from build123d import *

# Parameters (mm, degrees)
CROQUIS2_W                                = 104
CROQUIS2_H                                = 54
SALIENTE_EXTRUIR1_DEPTH                   = 66
CORTAR_EXTRUIR1_DEPTH                     = 36
TALADROS_DE_ESPIGA_DE_16_0MM1_D           = 16
TALADROS_DE_ESPIGA_DE_16_0MM1_DEPTH       = 36
TALADROS_DE_ESPIGA_DE_16_0MM1_CSINK_D     = 16.05
TALADROS_DE_ESPIGA_DE_16_0MM1_CSINK_ANGLE = 90
TALADROS_DE_ESPIGA_DE_16_0MM1_TIP         = 4.806884952
CROQUIS7_W                                = 28
CROQUIS7_H                                = 44
SALIENTE_EXTRUIR2_DEPTH                   = 4
CORTAR_EXTRUIR3_DEPTH                     = 100.879927913
CORTAR_EXTRUIR3_DEPTH_BACK                = 100.879927913
CORTAR_EXTRUIR4_DEPTH                     = 100.879927913
CORTAR_EXTRUIR4_DEPTH_BACK                = 100.879927913
CROQUIS9_R                                = 2
TALADRO_ROSCADO_M102_D                    = 8.5
TALADRO_ROSCADO_M102_DEPTH                = 27.5
TALADRO_ROSCADO_M102_CSINK_D              = 10.05
TALADRO_ROSCADO_M102_CSINK_ANGLE          = 90
TALADRO_ROSCADO_M102_TIP                  = 2.553657631


with BuildPart() as part:
    # Croquis2 → Saliente-Extruir1 (new body)
    with BuildSketch(Plane.XY):
        with Locations((0, 27)):
            Rectangle(CROQUIS2_W, CROQUIS2_H)
    extrude(amount=SALIENTE_EXTRUIR1_DEPTH)

    # Croquis3 → Cortar-Extruir1 (cut)
    with BuildSketch(Plane.XY):
        with BuildLine():
            Line((25, 29), (25, 18))
            Line((25, 18), (52, 18))
            Line((52, 18), (52, 54))
            Line((52, 54), (0, 54))
            ThreePointArc((0, 54), (17.67766953, 46.67766953), (25, 29))
        make_face()
    cortar_extruir1 = extrude(amount=CORTAR_EXTRUIR1_DEPTH, mode=Mode.SUBTRACT)

    # Simetría1: Cortar-Extruir1 across plane
    add(cortar_extruir1.mirror(Plane(origin=(0, 0, 0), x_dir=(0, 0, 1), z_dir=(1, 0, 0))), mode=Mode.SUBTRACT)

    # Taladros de espiga de Ø16.0mm1
    with Locations(Plane(origin=(0, 0, 0), x_dir=(-1, 0, 0), z_dir=(0, 0, -1))):
        with Locations((0, 28)):
            CounterSinkHole(TALADROS_DE_ESPIGA_DE_16_0MM1_D / 2, TALADROS_DE_ESPIGA_DE_16_0MM1_CSINK_D / 2, depth=TALADROS_DE_ESPIGA_DE_16_0MM1_DEPTH, counter_sink_angle=TALADROS_DE_ESPIGA_DE_16_0MM1_CSINK_ANGLE)
            with Locations((0, 0, -(TALADROS_DE_ESPIGA_DE_16_0MM1_DEPTH + TALADROS_DE_ESPIGA_DE_16_0MM1_TIP / 2))):  # 118° drill point
                Cone(0, TALADROS_DE_ESPIGA_DE_16_0MM1_D / 2, TALADROS_DE_ESPIGA_DE_16_0MM1_TIP, mode=Mode.SUBTRACT)

    # Croquis7 → Saliente-Extruir2 (add)
    with BuildSketch(Plane(origin=(0, 0, 0), x_dir=(1, 0, 0), z_dir=(0, 1, 0))):
        with Locations((0, -22)):
            Rectangle(CROQUIS7_W, CROQUIS7_H)
    extrude(amount=-SALIENTE_EXTRUIR2_DEPTH)

    # Croquis8 → Cortar-Extruir3 (cut, two sides: drawn at the far end of the back side and taken through both)
    with BuildSketch(Plane(origin=(0, 0, 0), x_dir=(0, 0, -1), z_dir=(1, 0, 0)).offset(-CORTAR_EXTRUIR3_DEPTH_BACK)):
        Polygon((-44, 0), (-56.494918643, 0), (-66, 0), (-66, 24), (-56, 24), (-56, 4), (-44, 4), align=None)
    extrude(amount=CORTAR_EXTRUIR3_DEPTH + CORTAR_EXTRUIR3_DEPTH_BACK, mode=Mode.SUBTRACT)

    # Croquis9 → Cortar-Extruir4 (cut, two sides: drawn at the far end of the back side and taken through both)
    with BuildSketch(Plane(origin=(0, 0, 0), x_dir=(0, 0, -1), z_dir=(1, 0, 0)).offset(-CORTAR_EXTRUIR4_DEPTH_BACK)):
        with Locations((-18, 29)):
            Circle(CROQUIS9_R)
    extrude(amount=CORTAR_EXTRUIR4_DEPTH + CORTAR_EXTRUIR4_DEPTH_BACK, mode=Mode.SUBTRACT)

    # Croquis13 → Taladro roscado M101 (revolve, cut)
    with BuildSketch(Plane(origin=(30, 44, 66), x_dir=(0, -1, 0), z_dir=(1, 0, 0))):
        Polygon((0, 0), (0, 11.553657631), (4.25, 9), (4.25, 0.775), (5.025, 0), align=None)
    taladro_roscado_m101 = revolve(axis=Axis((30, 44, 72.35), (0, 0, -1)), mode=Mode.SUBTRACT)

    # Simetría2: Taladro roscado M101 across plane
    add(taladro_roscado_m101.mirror(Plane.ZY), mode=Mode.SUBTRACT)

    # Taladro roscado M102
    with Locations(Plane(origin=(0, -4, 0), x_dir=(-1, 0, 0), z_dir=(0, -1, 0))):
        with Locations((0, -36), (0, -14)):
            CounterSinkHole(TALADRO_ROSCADO_M102_D / 2, TALADRO_ROSCADO_M102_CSINK_D / 2, depth=TALADRO_ROSCADO_M102_DEPTH, counter_sink_angle=TALADRO_ROSCADO_M102_CSINK_ANGLE)
            with Locations((0, 0, -(TALADRO_ROSCADO_M102_DEPTH + TALADRO_ROSCADO_M102_TIP / 2))):  # 118° drill point
                Cone(0, TALADRO_ROSCADO_M102_D / 2, TALADRO_ROSCADO_M102_TIP, mode=Mode.SUBTRACT)


solid = part.part
Check sheet for the modelled part. Datum: model origin and axes. Units: mm. A direction names the side the tool comes from. Give positions to 0.01 mm unless a question says otherwise; leave off trailing zeros. Write each loop counter-clockwise with the first axis right and the second up, starting at its lowest first coordinate (ties: lowest second). Pieces come first, ordered by that corner, then holes. Notation, with made-up numbers: M 16,-23 L 64,-23 A29 cw 64,5 Z; hole C 20,-26.5 d8. An arc over 180 degrees is marked long. Use one line per item in the form item = value.
(1) Section check D-D on x = 23.5. Record the boundary of the cut face in (y, z), plus the area to 3 significant figures.
Answer block:
outline = M 0,0 L 37.53,0 L 37.53,36 L 54,36 L 54,66 L 24,66 L 24,56 L 4,56 L 4,44 L 0,44 Z; hole C 29,18 d4
area = 2,670 mm2
(2) Tool access check on faces 4 (the cylindrical face through (-0.92, 10.32, 40.15)), 5 (the flat face through (37, 36, 36)), 6 (the flat face through (-37, 36, 36)), 7 (the flat face through (-1, 1, 44)), 8 (the flat face through (14, -2, 22)). Record the directions out of +Z, -Z, +X, -X, +Y, -Y that give a thin tool (end or side, any length) a straight path to the whole face; none if there is none.
Answer block:
face_4 = -Y
face_5 = -Z, +X, +Y
face_6 = -Z, -X, +Y
face_7 = +Z, +X, -X, -Y
face_8 = +Z, -Z, +X, -Y
(3) Draft check along Y on faces 1 (the cylindrical face through (16.085, 29.601, 16.092)), 2 (the flat face through (25, 24, 18)), 3 (the flat face through (38, 18, 18)). Enter one of: pulls with the +Y half, pulls with the -Y half, needs draft (parallel to the pull), parting line crosses it, or undercut.
Answer block:
face_1 = undercut
face_2 = needs draft
face_3 = pulls with the +Y half
(4) Section check C-C on y = 7.5. Record the boundary of the cut face in (x, z), plus the area to 3 significant figures.
Answer block:
outline = M -52,0 L 52,0 L 52,56 L -52,56 Z; hole C 0,14 d8.5; hole C 0,36 d8.5
area = 5,710 mm2
(5) Depth check by flat-ended pin: P1, Ø5, axis at y = 29, z = 18, coming from the -X side; P2, Ø4.5, axis at y = -3, z = 11.5, coming from the +X side; P3, Ø1.2, axis at y = -1.5, z = 17, coming from the -X side. Enter the tip coordinate at first touch or a pass-through.
Answer block:
P1 = -25
P2 = 14
P3 = -14
(6) Section check A-A on x = -45. Record the boundary of the cut face in (y, z).
Answer block:
outline = M 0,0 L 18,0 L 18,36 L 54,36 L 54,66 L 24,66 L 24,56 L 4,56 L 4,44 L 0,44 Z
(7) Section check B-B on z = 14. Record the boundary of the cut face in (x, y) (3 decimals).
Answer block:
outline = M -52,0 L -14,0 L -14,-4 L -5.025,-4 L -4.25,-3.225 L -4.25,21.222 A8 cw long 4.25,21.222 L 4.25,-3.225 L 5.025,-4 L 14,-4 L 14,0 L 52,0 L 52,18 L 25,18 L 25,29 A25 ccw -25,29 L -25,18 L -52,18 Z
(8) Material ranges on line 1 along X through (y, z) = (44, 60.25); line 2 along X through (y, z) = (6, 36); line 3 along Z through (x, y) = (25, 37), recorded low to high.
Answer block:
line_1 = -52 to -34.25, -25.75 to 25.75, 34.25 to 52
line_2 = -52 to -4.25, 4.25 to 52
line_3 = 36 to 66
